Input: part model. Units: mm. Frame: model coordinates. Give positions to 0.01 mm unless a question says otherwise; leave off trailing zeros. Order: outer loops, then holes, each group sorted by start corner. A loop starts at its lowest first (then second) coordinate and runs counter-clockwise, first axis right, second up. Notation, with made-up numbers: (-33, 61) - (-15, 61) arc R19 ccw to (-15, 94) - close; hole circle Ø11 at (8.5, 16). An arc over 180 degrees is marked (long way). Use a Markdown table: item, result.
from build123d import *

# Parameters (mm, degrees)
EXTRUDE_1_DEPTH     = 20
SKETCH_1_3_W        = 2.5
SKETCH_1_3_H        = 401
SKETCH_2_R          = 2.5
CUT_EXTRUDE_1_DEPTH = 447.597133891


with BuildPart() as part:
    # Sketch 1 → Extrude 1 (new, symmetric)
    with BuildSketch(Plane.XY):
        Polygon((17.5, -42), (22.5, -42), (40, -42), (40, 0), (0, 0), (0, -42), align=None)
    extrude(amount=EXTRUDE_1_DEPTH, both=True)

    # Sketch 1_3 → Revolve 1 (revolve)
    with BuildSketch(Plane.XY, mode=Mode.PRIVATE) as revolve_1_sk:
        with Locations((21.25, -242.5)):
            Rectangle(SKETCH_1_3_W, SKETCH_1_3_H)
    revolve(revolve_1_sk.sketch.rotate(Axis((20, -42, 0), (0, -1, 0)), 180), axis=Axis((20, -42, 0), (0, -1, 0)))

    # Sketch 2 → Cut-Extrude 1 (cut, through all)
    with BuildSketch(Plane.XY.offset(20)):
        with Locations((6.5, -35.5)):
            Circle(SKETCH_2_R)
        with Locations((33.5, -35.5)):
            Circle(SKETCH_2_R)
    extrude(amount=-CUT_EXTRUDE_1_DEPTH, mode=Mode.SUBTRACT)


solid = part.part
1. Section query A-A (z = 16). Return loops of the section in (x, y).
Response:
| item | result |
|---|---|
| outline | (0, -42) - (40, -42) - (40, 0) - (0, 0) - close; hole circle Ø5 at (6.5, -35.5); hole circle Ø5 at (33.5, -35.5) |
2. Material intervals for line 1 along X through (y, z) = (-35, 10); line 2 along Y through (x, z) = (33.5, -11); line 3 along Y through (x, z) = (33, 4), sorted ascending.
Response:
| item | result |
|---|---|
| line 1 | x = 0 to 4.05, 8.95 to 31.05, 35.95 to 40 |
| line 2 | y = -42 to -38, -33 to 0 |
| line 3 | y = -42 to -37.95, -33.05 to 0 |
3. Pin query (flat end, axial travel): pin 1 (12 mm diameter, centred on x = 29, z = -7.5, fed in from +Y); pin 2 (10 mm diameter, centred on x = 26, z = -5, fed in from -Y). Return the tip coordinate at first contact, or that it passes through.
Response:
| item | result |
|---|---|
| pin 1 | stops at y = 0 |
| pin 2 | stops at y = -42 |
4. Section query B-B (y = -173). Return loops of the section in (x, z).
Response:
| item | result |
|---|---|
| outline | circle Ø5 at (20, 0) |
